Part model, mm, in its own coordinate system. Coordinates: 2 decimals unless noted, no trailing zeros. Loops run counter-clockwise (first coordinate to the right, second up) from the corner with the lowest first, then second, coordinate; pieces in that order, holes last. Notation, with made-up numbers: (-16.5, 73) - (16.5, 73) arc R17 cw to (16.5, 91) - close; hole circle Ø10 at (23.5, -20.75). An arc over 180 degrees is marked (long way). Answer as CSV lines item,"result".
from build123d import *

# Parameters (mm, degrees)
F0_W     = 127
F0_H     = 76.2
F1_DEPTH = 76.2
F3_DEPTH = 127.001
F4_R     = 25.4


with BuildPart() as f1:
    # F0 (on Front) → F1 (new body)
    with BuildSketch(Plane.XZ):
        Rectangle(F0_W, F0_H)
    extrude(amount=F1_DEPTH)

    # F2 (on face) → F3 (cut, through all)
    with BuildSketch(Plane(origin=(-63.5, 0, 0), x_dir=(0, -1, 0), z_dir=(-1, 0, 0))):
        with BuildLine():
            ThreePointArc((14.3655382942, 38.1), (37.6635127669, 61.5633803993), (68.9486063382, 72.2670598849))
            Line((68.9486063382, 72.2670598849), (-52.0951251411, 60.1213361119))
            Line((-52.0951251411, 60.1213361119), (-33.0926589668, -48.5322624445))
            Line((-33.0926589668, -48.5322624445), (48.5539544729, -67.162540312))
            ThreePointArc((48.5539544729, -67.162540312), (29.1590805148, -55.3377136177), (14.3655382942, -38.1))
            Line((14.3655382942, -38.1), (0, -38.1))
            Line((0, -38.1), (0, 38.1))
            Line((0, 38.1), (14.3655382942, 38.1))
        make_face()
        with BuildLine():
            ThreePointArc((14.3655382942, -38.1), (3.5700429957, 0), (14.3655382942, 38.1))
            Line((14.3655382942, 38.1), (0, 38.1))
            Line((0, 38.1), (0, -38.1))
            Line((0, -38.1), (14.3655382942, -38.1))
        make_face()
    extrude(amount=-F3_DEPTH, mode=Mode.SUBTRACT)

    # F4
    f4_edges = [f1.edges().sort_by_distance(p)[0] for p in [
        (-63.5, -45.282769, 38.1),
        (63.5, -45.282769, 38.1),
        (-63.5, -45.282769, -38.1),
        (63.5, -45.282769, -38.1),
        (63.5, -3.570043, 0),
        (-63.5, -3.570043, 0),
        (0, -14.365538, -38.1),
        (0, -14.365538, 38.1),
    ]]
    fillet(f4_edges, radius=F4_R)


solid = f1.part
Q1. Wall check: L1, parallel to X at y = -69.5, z = -13.5; L2, parallel to Z at x = 46.5, y = -45.5; L3, parallel to Z at x = -41, y = -26.5. Give the ranges that are in metal, low to high.
Results:
L1,"x = -63.49 to 63.49"
L2,"z = -36.67 to 36.67"
L3,"z = -37.58 to 37.58"
Q2. Saw through at C-C (z = 31). Give the cut face in (x, y).
Results:
outline,"(-55.71, -76.2) - (55.71, -76.2) - (55.71, -30.71) arc R17.61 ccw to (38.1, -13.1) - (-38.1, -13.1) arc R17.61 ccw to (-55.71, -30.71) - close"
Q3. Saw through at A-A (x = -30). Give the cut face in (y, z), then the cut area to 3 significant figures.
Results:
outline,"(-76.2, -38.1) - (-30.71, -38.1) arc R25.4 ccw to (-6.25, -19.53) arc R72.63 ccw to (-6.25, 19.53) arc R25.4 ccw to (-30.71, 38.1) - (-76.2, 38.1) - close"
area,"5,160 mm^2"
Q4. Saw through at B-B (y = -56). Give the cut face in (x, z).
Results:
outline,"(-63.5, -12.7) arc R25.4 ccw to (-38.1, -38.1) - (38.1, -38.1) arc R25.4 ccw to (63.5, -12.7) - (63.5, 12.7) arc R25.4 ccw to (38.1, 38.1) - (-38.1, 38.1) arc R25.4 ccw to (-63.5, 12.7) - close"
Q5. Flat gauge pins, fed straight in: pin 1 (5 mm diameter, centred on y = -57.5, z = -15.5, fed in from -X); pin 2 (6 mm diameter, centred on x = 39.5, z = -5.5, fed in from +Y); pin 3 (1 mm diameter, centred on x = -23, z = 15.5, fed in from +Y). Where does each tip first touch, or does it go through?
Results:
pin 1,"stops at x = -63.5"
pin 2,"stops at y = -3.62"
pin 3,"stops at y = -5.14"
